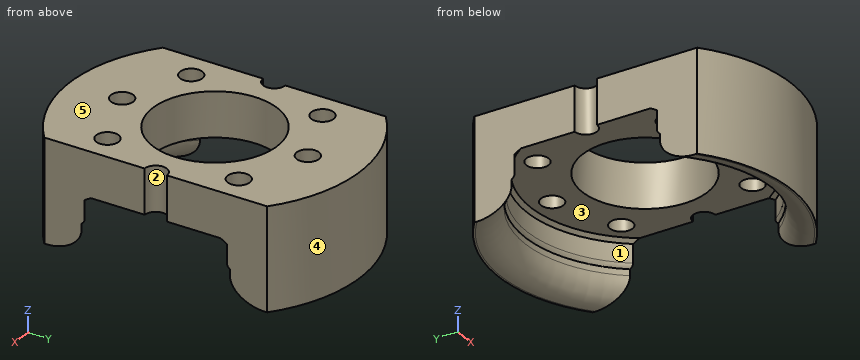
from build123d import *

# Parameters (mm, degrees)
BOSS_EXTRUDE1_OUTLINE_R     = 39.0639683
BOSS_EXTRUDE1_OUTLINE_R_2   = 3
BOSS_EXTRUDE1_OUTLINE_R_3   = 16.75
BOSS_EXTRUDE1_DEPTH         = 12
BOSS_EXTRUDE1_START         = -9.0000001
BOSS_EXTRUDE1_2_OUTLINE_R   = 39.0639683
BOSS_EXTRUDE1_2_OUTLINE_R_2 = 32
BOSS_EXTRUDE1_2_DEPTH       = 9.0000001
BOSS_EXTRUDE1_START_2       = -6.0000001
BOSS_EXTRUDE1_3_OUTLINE_R   = 32
BOSS_EXTRUDE1_3_OUTLINE_R_2 = 31.5
BOSS_EXTRUDE1_3_DEPTH       = 6.0000001
CUT_EXTRUDE1_REACH          = 63.711


with BuildPart() as part:
    # Boss-Extrude1: read off the stored shape, not the designer's step
    # Boss-Extrude1 outline → Boss-Extrude1 (new body)
    with BuildSketch(Plane.XY):
        Circle(BOSS_EXTRUDE1_OUTLINE_R)
        with Locations((0, 25)):
            Circle(BOSS_EXTRUDE1_OUTLINE_R_2, mode=Mode.SUBTRACT)
        with Locations((-17.67766953, -17.67766953)):
            Circle(BOSS_EXTRUDE1_OUTLINE_R_2, mode=Mode.SUBTRACT)
        with Locations((0, -25)):
            Circle(BOSS_EXTRUDE1_OUTLINE_R_2, mode=Mode.SUBTRACT)
        with Locations((17.67766953, -17.67766953)):
            Circle(BOSS_EXTRUDE1_OUTLINE_R_2, mode=Mode.SUBTRACT)
        with Locations((-25, 0)):
            Circle(BOSS_EXTRUDE1_OUTLINE_R_2, mode=Mode.SUBTRACT)
        with Locations((-17.67766953, 17.67766953)):
            Circle(BOSS_EXTRUDE1_OUTLINE_R_2, mode=Mode.SUBTRACT)
        Circle(BOSS_EXTRUDE1_OUTLINE_R_3, mode=Mode.SUBTRACT)
        with Locations((17.67766953, 17.67766953)):
            Circle(BOSS_EXTRUDE1_OUTLINE_R_2, mode=Mode.SUBTRACT)
        with Locations((25, 0)):
            Circle(BOSS_EXTRUDE1_OUTLINE_R_2, mode=Mode.SUBTRACT)
    extrude(amount=BOSS_EXTRUDE1_DEPTH)



with BuildPart() as body_2:
    # Boss-Extrude1 2 outline → Boss-Extrude1 2 (new body)
    with BuildSketch(Plane.XY.offset(BOSS_EXTRUDE1_START)):
        Circle(BOSS_EXTRUDE1_2_OUTLINE_R)
        Circle(BOSS_EXTRUDE1_2_OUTLINE_R_2, mode=Mode.SUBTRACT)
    extrude(amount=BOSS_EXTRUDE1_2_DEPTH)


with BuildPart() as body_3:
    # Boss-Extrude1 3 outline → Boss-Extrude1 3 (new body)
    with BuildSketch(Plane.XY.offset(BOSS_EXTRUDE1_START_2)):
        Circle(BOSS_EXTRUDE1_3_OUTLINE_R)
        Circle(BOSS_EXTRUDE1_3_OUTLINE_R_2, mode=Mode.SUBTRACT)
    extrude(amount=BOSS_EXTRUDE1_3_DEPTH)


with BuildPart() as part_1:
    add(part.part)

    add(body_2.part)  # Boss-Extrude1 4 merges body 2

    add(body_3.part)  # Boss-Extrude1 4 merges body 3
    # Boss-Extrude1 4 outline → Boss-Extrude1 4 (revolve)
    with BuildSketch(Plane.XZ):
        Polygon((31.499999999, -1.000000001), (31.499999999, 0), (30.5, 0), align=None)
        with BuildLine():
            Line((32, -7.322875656), (32, -6.0000001))
            Line((32, -6.0000001), (31.5, -6))
            ThreePointArc((31.5, -6), (31.629171307, -6.707106781), (32, -7.322875656))
        make_face()
        with BuildLine():
            Line((39.0639683, -15.5), (39.0639683, -9.0000001))
            Line((39.0639683, -9.0000001), (32, -9))
            ThreePointArc((32, -9), (33.903805922, -13.596194078), (38.5, -15.5))
            Line((38.5, -15.5), (39.0639683, -15.5))
        make_face()
    revolve(axis=Axis((0, 0, 0), (0, 0, 1)))

    # Sketch2 → Cut-Extrude1 (cut, up to next)
    with BuildSketch(Plane.XY.offset(12), mode=Mode.PRIVATE) as cut_extrude1_sk1:
        with BuildLine():
            Line((-25, -30.016555754), (-25, 30.016555754))
            ThreePointArc((-25, 30.016555754), (-39.0639683, 0), (-25, -30.016555754))
        make_face()
    cut_extrude1_tool1 = extrude(cut_extrude1_sk1.sketch, amount=-CUT_EXTRUDE1_REACH, mode=Mode.PRIVATE) & part_1.part
    # Sketch2 → Cut-Extrude1 (cut, up to next)
    with BuildSketch(Plane.XY.offset(12), mode=Mode.PRIVATE) as cut_extrude1_sk2:
        with BuildLine():
            Line((25, -30.016555754), (25, 30.016555754))
            ThreePointArc((25, 30.016555754), (39.0639683, 0), (25, -30.016555754))
        make_face()
    cut_extrude1_tool2 = extrude(cut_extrude1_sk2.sketch, amount=-CUT_EXTRUDE1_REACH, mode=Mode.PRIVATE) & part_1.part
    add(cut_extrude1_tool1.solids().sort_by_distance((-30.722563, 0, 12))[0], mode=Mode.SUBTRACT)
    add(cut_extrude1_tool2.solids().sort_by_distance((30.722563, 0, 12))[0], mode=Mode.SUBTRACT)


solid = part_1.part
Design review of the part built by this model. Coordinates are the model's own, in mm. Face numbers are marked on the shaded views. A direction names the side the tool comes from. Coordinates: 2 decimals unless noted, no trailing zeros. Order: outer loops, then holes, each group sorted by start corner. A loop starts at its lowest first (then second) coordinate and runs counter-clockwise, first axis right, second up. Notation, with made-up numbers: M 77.25,85 L 125.25,85 A21 cw 125.25,97 Z; hole C 77.5,-29 d1. An arc over 180 degrees is marked long. Use a Markdown table: item, result.
(1) Draft analysis for pull direction X (two halves, no side actions). For the marked faces 3, 4 and 5, state which applies: released by +X, released by -X, zero draft, split by the parting line, or undercut.
Worked answers:
| item | result |
|---|---|
| face 3 | undercut |
| face 4 | split by the parting line |
| face 5 | zero draft |
(2) Wall thickness on probe 1 along Y at (x, z) = (0, 9.25); probe 2 along Y at (x, z) = (17, 8.5); probe 3 along Y at (x, z) = (1, -8.5): over which ranges is each line inside the solid? List them lowest first.
Worked answers:
| item | result |
|---|---|
| probe 1 | y = -39.06 to -28, -22 to -16.75, 16.75 to 22, 28 to 39.06 |
| probe 2 | y = -35.17 to -20.6, -14.76 to 14.76, 20.6 to 35.17 |
| probe 3 | y = -39.05 to -31.98, 31.98 to 39.05 |
(3) For the marked faces 1 and 2, list the 3-axis set-ups (+Z, -Z, +X, -X, +Y, -Y) from which the entire face can be reached by the end or side of a thin tool; tool diameter is ignored.
Worked answers:
| item | result |
|---|---|
| face 1 | -Z |
| face 2 | +Z, -Z, +X |
(4) For P1, Ø5.5, axis at x = 17.68, y = -17.68, coming from the +Z side; P2, Ø10, axis at y = 11, z = -2.5, coming from the +X side; P3, Ø2, axis at x = -4.5, z = 7.5, coming from the +Y side; P4, Ø2, axis at x = 3, z = -9, coming from the +Y side, all flat-tipped, find the tip position at first contact; note any pin that passes through.
Worked answers:
| item | result |
|---|---|
| P1 | passes through |
| P2 | stops at x = 25 |
| P3 | stops at y = 38.91 |
| P4 | stops at y = 39.01 |
(5) Add section C-C (y = 15.5). Give the boundary of the cut face in (x, z).
Worked answers:
| item | result |
|---|---|
| outline | M -25,0 L -19.74,0 L -19.74,12 L -25,12 Z; M -15.61,0 L -6.35,0 L -6.35,12 L -15.61,12 Z; M 6.35,0 L 15.61,0 L 15.61,12 L 6.35,12 Z; M 19.74,0 L 25,0 L 25,12 L 19.74,12 Z |
(6) Add section D-D (z = -14). Give the boundary of the cut face in (x, y), then the cut area to 3 significant figures.
Worked answers:
| item | result |
|---|---|
| outline | M -25,-30.02 A39.06 ccw 25,-30.02 L 25,-23.55 A34.35 cw -25,-23.55 Z; M -25,23.55 A34.35 cw 25,23.55 L 25,30.02 A39.06 ccw -25,30.02 Z |
| area | 519 mm2 |
(7) Add section B-B (x = 0). Give the boundary of the cut face in (y, z).
Worked answers:
| item | result |
|---|---|
| outline | M -39.06,-15.5 L -38.5,-15.5 A6.5 ccw -32,-9 L -32,-7.32 A2 ccw -31.5,-6 L -31.5,-1 L -30.5,0 L -28,0 L -28,12 L -39.06,12 Z; M -22,0 L -16.75,0 L -16.75,12 L -22,12 Z; M 16.75,0 L 22,0 L 22,12 L 16.75,12 Z; M 28,0 L 30.5,0 L 31.5,-1 L 31.5,-6 A2 ccw 32,-7.32 L 32,-9 A6.5 ccw 38.5,-15.5 L 39.06,-15.5 L 39.06,12 L 28,12 Z |
(8) Add section A-A (z = -2.25). Give the boundary of the cut face in (x, y), then the cut area to 3 significant figures.
Worked answers:
| item | result |
|---|---|
| outline | M -25,-30.02 A39.06 ccw 25,-30.02 L 25,-19.16 A31.5 cw -25,-19.16 Z; M -25,19.16 A31.5 cw 25,19.16 L 25,30.02 A39.06 ccw -25,30.02 Z |
| area | 843 mm2 |
